The listing builds one solid part. Answer for the finished solid, in the listing's coordinates (mm). Face numbers are marked on the shaded views. A direction names the side the tool comes from. Coordinates: 2 decimals unless noted, no trailing zeros. Loops run counter-clockwise (first coordinate to the right, second up) from the corner with the lowest first, then second, coordinate; pieces in that order, holes last. Notation, with made-up numbers: (57.25, -15) - (84.25, -15) arc R18 ccw to (84.25, 0) - close; hole circle Ø8 at (-34.75, -8.5). An arc over 180 degrees is marked (long way). Put each result on its own line as item: value.
Autodesk Inventor part; units mm, degrees
ref_plane "YZ Plane" through (0, 0, 0) normal (1, 0, 0) x (0, 1, 0)
ref_plane "XZ Plane" through (0, 0, 0) normal (0, 1, 0) x (-1, 0, 0)
ref_plane "XY Plane" through (0, 0, 0) normal (0, 0, 1) x (1, 0, 0)
sketch "Skizze1" plane through (0, 0, 0) normal (0, 1, 0) x (-1, 0, 0)
  line L0 (0, 16) -> (0, 0)
  line L1 (0, 16) -> (-0.6, 16)
  line L2 (-0.6, 16) -> (-0.6, 9)
  line L3 (0, 0) -> (-0.6, 0)
  line L4 (0, 0) -> (0.6, 0) construction
  line L5 (-0.6, 0) -> (-0.6, 6)
  line L6 (-4.2, 6) -> (-3.2, 6)
  line L7 (-3.2, 6) -> (-3.2, 6.5)
  arc A0 (-1.7, 6.5) -> (-3.2, 6.5) centre (-2.45, 6.5) ccw
  line L8 (-1.7, 6.5) -> (-1.7, 6)
  line L9 (-1.7, 6) -> (-0.6, 6)
  line L10 (-11.5, 23.3819) -> (-11.5, -15) construction
  line L11 (-4.2, 6) -> (-4.2, 0)
  line L12 (-4.2, 0) -> (-4.8, 0)
  line L13 (-4.8, 0) -> (-4.8, 8)
  line L14 (-4.8, 8) -> (-8.5, 8)
  line L15 (-0.6, 9) -> (-11.5, 9)
  line L16 (-8.5, 8) -> (-8.5, 0)
  line L17 (-8.5, 0) -> (-9.1, 0)
  line L18 (-9.1, 0) -> (-9.1, 6.7)
  line L19 (-9.1, 6.7) -> (-11.5, 6.7)
  line L20 (-23, 16) -> (-23, 0)
  line L21 (-23, 16) -> (-22.4, 16)
  line L22 (-22.4, 16) -> (-22.4, 9)
  line L23 (-23, 0) -> (-22.4, 0)
  line L24 (-23, 0) -> (-23.6, 0) construction
  line L25 (-22.4, 0) -> (-22.4, 6)
  line L26 (-19.8, 6) -> (-19.8, 6.5)
  line L27 (-18.8, 6) -> (-19.8, 6)
  arc A1 (-19.8, 6.5) -> (-21.3, 6.5) centre (-20.55, 6.5) ccw
  line L28 (-21.3, 6.5) -> (-21.3, 6)
  line L29 (-21.3, 6) -> (-22.4, 6)
  line L30 (-18.8, 6) -> (-18.8, 0)
  line L31 (-18.8, 0) -> (-18.2, 0)
  line L32 (-18.2, 0) -> (-18.2, 8)
  line L33 (-18.2, 8) -> (-14.5, 8)
  line L34 (-22.4, 9) -> (-11.5, 9)
  line L35 (-14.5, 8) -> (-14.5, 0)
  line L36 (-14.5, 0) -> (-13.9, 0)
  line L37 (-13.9, 0) -> (-13.9, 6.7)
  line L38 (-13.9, 6.7) -> (-11.5, 6.7)
  point P0 (0, 0)
  point P1 (-23, 0)
  dimension "d0" = 16
  dimension "d1" = 0.6
  dimension "d2" = 7
  dimension "d22" = 0.6
  dimension "d24" = 6
  dimension "d25" = 1
  dimension "d26" = 0.5
  dimension "d27" = 90
  dimension "d28" = 1.1
  dimension "d29" = 0.75
  dimension "d30" = 1.25
  dimension "d31" = 1.25
  dimension "d32" = 1.5
  dimension "d37" = 0.6
  dimension "d38" = 8
  dimension "d39" = 3.7
  dimension "d40" = 23
  dimension "d41" = 0.6
  dimension "d42" = 6.7
  dimension "d43" = 2.3
extrude "Extrusion1" add sketch "Skizze1" along normal blind 25
sketch "Skizze2" plane through (13.9, 0, 6.7) normal (0, 0, -1) x (-1, 0, 0)
  line L0 (0, 25) -> (4.8, 25)
  line L1 (0, 0) -> (0, 25)
  point P0 (13.9, 0)
  point P1 (2.4, 18)
  dimension "d46" = 7
  dimension "d47" = 2.4
hole "Bohrung1" at (11.5, 18, 6.7) direction (0, 0, 1) diameter 3 end through all
properties part number "Kühlkörper"
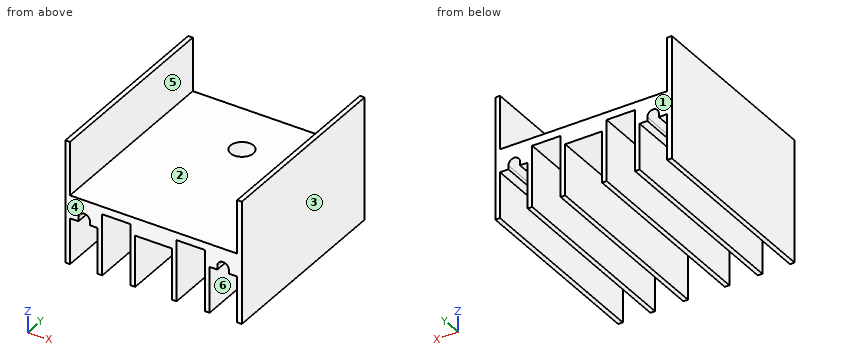
1) The part is cut by section D-D (x = 7). Give the vertices of the cut face in (y, z), and give its area (3 significant figures).
Found:
outline: (0, 8) - (25, 8) - (25, 9) - (0, 9) - close
area: 25.0 mm^2
2) Each of these flat-tipped pins is pushed along its axis until it touches: pin 1 (3.5 mm diameter, centred on x = 11.5, y = 18, fed in from +Z); pin 2 (1.5 mm diameter, centred on x = 6.5, z = 11, fed in from +Y). Where does it stop, or does it pass through?
Found:
pin 1: stops at z = 9
pin 2: passes through
3) Straight lines are drawn through the part: L1, parallel to X at y = 18, z = 7.3; L2, parallel to X at y = 8, z = 4.25; L3, parallel to X at y = 18, z = 8.4. For each, find the intervals that lie inside material, in ascending order. Write a range as [from, to].
Found:
L1: x = [0, 4.8], [8.5, 10], [13, 14.5], [18.2, 23]
L2: x = [0, 0.6], [4.2, 4.8], [8.5, 9.1], [13.9, 14.5], [18.2, 18.8], [22.4, 23]
L3: x = [0, 10], [13, 23]
4) The part is cut by section A-A (z = 4.75). Give the vertices of the cut face in (x, y).
Found:
outline: (0, 0) - (0.6, 0) - (0.6, 25) - (0, 25) - close; (4.2, 0) - (4.8, 0) - (4.8, 25) - (4.2, 25) - close; (8.5, 0) - (9.1, 0) - (9.1, 25) - (8.5, 25) - close; (13.9, 0) - (14.5, 0) - (14.5, 25) - (13.9, 25) - close; (18.2, 0) - (18.8, 0) - (18.8, 25) - (18.2, 25) - close; (22.4, 0) - (23, 0) - (23, 25) - (22.4, 25) - close
5) For a pull along X with two mould halves and no side action, classify the marked faces 1, 2 and 3 as pulls with the +X half, pulls with the -X half, needs draft (parallel to the pull), parting line crosses it, or undercut.
Found:
face 1: needs draft
face 2: undercut
face 3: pulls with the +X half
6) For the marked faces 4, 5 and 6, determine the directions among +Z, -Z, +X, -X, +Y, -Y from which every point of the face is accessible in a straight line to the end or side of a thin tool.
Found:
face 4: +Z, -Z, +X, -X, -Y
face 5: +Z, +Y, -Y
face 6: -Z, +Y, -Y
7) The part is cut by section C-C (z = 15). Give the vertices of the cut face in (x, y), and give its area (3 significant figures).
Found:
outline: (0, 0) - (0.6, 0) - (0.6, 25) - (0, 25) - close; (22.4, 0) - (23, 0) - (23, 25) - (22.4, 25) - close
area: 30.0 mm^2
8) The part is cut by section B-B (x = 11.5). Give the vertices of the cut face in (y, z), and give its area (3 significant figures).
Found:
outline: (0, 6.7) - (16.5, 6.7) - (16.5, 9) - (0, 9) - close; (19.5, 6.7) - (25, 6.7) - (25, 9) - (19.5, 9) - close
area: 50.6 mm^2
